```python
from build123d import *

# Parameters (mm, degrees)
SKETCH2_W           = 45
SKETCH2_H           = 10
BOSS_EXTRUDE1_DEPTH = 40
SKETCH4_W           = 45
SKETCH4_H           = 10
BOSS_EXTRUDE2_DEPTH = 10
SKETCH8_W           = 45
SKETCH8_H           = 10
BOSS_EXTRUDE3_DEPTH = 20
SKETCH9_R           = 1.45
CUT_EXTRUDE2_DEPTH  = 20
SKETCH10_W          = 45
SKETCH10_H          = 0.626165357
CUT_EXTRUDE3_DEPTH  = 2
SKETCH11_W          = 19
SKETCH11_H          = 42.671327575
BOSS_EXTRUDE4_DEPTH = 1.5
SKETCH12_W          = 3
SKETCH12_H          = 27.286335608
CUT_EXTRUDE6_DEPTH  = 10


with BuildPart() as part:
    # Sketch2 → Boss-Extrude1 (new body)
    with BuildSketch(Plane(origin=(0, 0, 0), x_dir=(1, 0, 0), z_dir=(0, 1, 0))):
        Rectangle(SKETCH2_W, SKETCH2_H)
    extrude(amount=BOSS_EXTRUDE1_DEPTH)

    # Sketch4 → Boss-Extrude2 (add)
    with BuildSketch(Plane(origin=(0, 40, 0), x_dir=(1, 0, 0), z_dir=(0, 1, 0))):
        Rectangle(SKETCH4_W, SKETCH4_H)
    extrude(amount=BOSS_EXTRUDE2_DEPTH)

    # Sketch8 → Boss-Extrude3 (add)
    with BuildSketch(Plane.XZ):
        Rectangle(SKETCH8_W, SKETCH8_H)
    extrude(amount=BOSS_EXTRUDE3_DEPTH)

    # Sketch9 → Cut-Extrude2 (cut)
    with BuildSketch(Plane.XY.offset(5)):
        with Locations((19.5, 11.5)):
            Circle(SKETCH9_R)
        with Locations((-19.5, 11.5)):
            Circle(SKETCH9_R)
    extrude(amount=-CUT_EXTRUDE2_DEPTH, mode=Mode.SUBTRACT)

    # Sketch10 → Cut-Extrude3 (cut)
    with BuildSketch(Plane.XY.offset(5)):
        with Locations((0, 22.984410254)):
            Rectangle(SKETCH10_W, SKETCH10_H)
    extrude(amount=-CUT_EXTRUDE3_DEPTH, mode=Mode.SUBTRACT)

    # Sketch11 → Boss-Extrude4 (add)
    with BuildSketch(Plane.XY.offset(5)):
        with Locations((0, 1.335663788)):
            Rectangle(SKETCH11_W, SKETCH11_H)
    extrude(amount=BOSS_EXTRUDE4_DEPTH)

    # Sketch12 → Cut-Extrude6 (cut)
    with BuildSketch(Plane(origin=(22.5, 0, 0), x_dir=(0, 0, -1), z_dir=(1, 0, 0))):
        with Locations((0, -4.971840229)):
            Rectangle(SKETCH12_W, SKETCH12_H)
    cut_extrude6 = extrude(amount=-CUT_EXTRUDE6_DEPTH, mode=Mode.SUBTRACT)

    # Mirror1: Cut-Extrude6 across plane
    add(cut_extrude6.mirror(Plane(origin=(0, 0, 0), x_dir=(0, 0, 1), z_dir=(1, 0, 0))), mode=Mode.SUBTRACT)


solid = part.part
```
Verification items for the finished model (mm, model axes). A direction names the side the tool comes from. Give positions to 0.01 mm unless a question says otherwise; leave off trailing zeros. Order: outer loops, then holes, each group sorted by start corner. A loop starts at its lowest first (then second) coordinate and runs counter-clockwise, first axis right, second up. Notation, with made-up numbers: M 42.5,-35 L 90.5,-35 A10 ccw 90.5,-31 Z; hole C 89,-28.75 d6. An arc over 180 degrees is marked long. Return JSON: item names as keys, results as strings. Group by question number.
1) Mould release check, pull along Z, two halves, no side actions. Record for faces 1 (the face through (-18, 8.671, 0)), 2 (the face through (12.5, -5, 0)), 3 (the face through (-22.5, 15, 0)), 4 (the face through (0, 2, 6.5)): pulls with the +Z half, pulls with the -Z half, needs draft (parallel to the pull), parting line crosses it, or undercut.
2) Go/stop test with flat-tipped pins: pin 1 Ø0.8 at (y, z) = (6.5, 5.5) entering from -X; pin 2 Ø11 at (x, y) = (15.5, 1) entering from +Z; pin 3 Ø0.5 at (x, y) = (-5.5, 23) entering from +Z. Record where each tip stops, or that it passes through.
3) Scan lines: line 1 (Y direction, x = 19.5, z = 1.25) (3 decimals); line 2 (Y direction, x = 19.5, z = 3.25); line 3 (Y direction, x = -18, z = 4). Record each from-to range of solid material in increasing order.
4) Access from +Z, -Z, +X, -X, +Y, -Y to the whole of each face (thin tool, end or side, straight path). Record for faces 5 (the face through (18, 8.671, 0)), 6 (the face through (0, 23.297, 4)), 7 (the face through (-18, -5, 1.5)), 8 (the face through (0, 37, 5)).
5) Section check A-A on x = 19.5. Give the number of separate pieces and of enclosed holes in the cut face, and give its area (3 significant figures).
6) Section check B-B on y = 11.5. Record the cut outline in (x, z).
7) Section check D-D on y = 4.5. Record the cut outline in (x, z).
8) Section check C-C on x = -6.5. Record the cut outline in (y, z), and give its area (3 significant figures).
Answer block:
{
 "1": {"face 1": "undercut", "face 2": "undercut", "face 3": "needs draft", "face 4": "pulls with the +Z half"},
 "2": {"pin 1": "stops at x = -9.5", "pin 2": "stops at z = 5", "pin 3": "stops at z = 3"},
 "3": {"line 1": "y = -20 to -18.615, 8.671 to 10.05, 12.95 to 50", "line 2": "y = -20 to 10.05, 12.95 to 22.67, 23.3 to 50", "line 3": "y = -20 to 22.67, 23.3 to 50"},
 "4": {"face 5": "+X", "face 6": "+Z, +X, -X", "face 7": "-X", "face 8": "+Z, +X, -X, +Y"},
 "5": {"separate pieces": "2", "enclosed holes": "1", "area": "588 mm^2"},
 "6": {"outline": "M -22.5,-5 L -20.95,-5 L -20.95,5 L -22.5,5 Z; M -18.05,-5 L 18.05,-5 L 18.05,5 L 9.5,5 L 9.5,6.5 L -9.5,6.5 L -9.5,5 L -18.05,5 Z; M 20.95,-5 L 22.5,-5 L 22.5,5 L 20.95,5 Z"},
 "7": {"outline": "M -22.5,-5 L 22.5,-5 L 22.5,-1.5 L 12.5,-1.5 L 12.5,1.5 L 22.5,1.5 L 22.5,5 L 9.5,5 L 9.5,6.5 L -9.5,6.5 L -9.5,5 L -22.5,5 L -22.5,1.5 L -12.5,1.5 L -12.5,-1.5 L -22.5,-1.5 Z"},
 "8": {"outline": "M -20,-5 L 50,-5 L 50,5 L 23.3,5 L 23.3,3 L 22.67,3 L 22.67,6.5 L -20,6.5 Z", "area": "763 mm^2"}
}
